Design review of the part built by this model. Coordinates are the model's own, in mm. Coordinates: 2 decimals unless noted, no trailing zeros. Loops run counter-clockwise (first coordinate to the right, second up) from the corner with the lowest first, then second, coordinate; pieces in that order, holes last. Notation, with made-up numbers: (-7.75, -32.75) -> (23.25, -32.75) arc R22 cw to (23.25, 5.25) -> close; hole circle Ø3 at (-12, 18.5). An arc over 180 degrees is marked (long way). Answer in a Markdown table with one row per item.
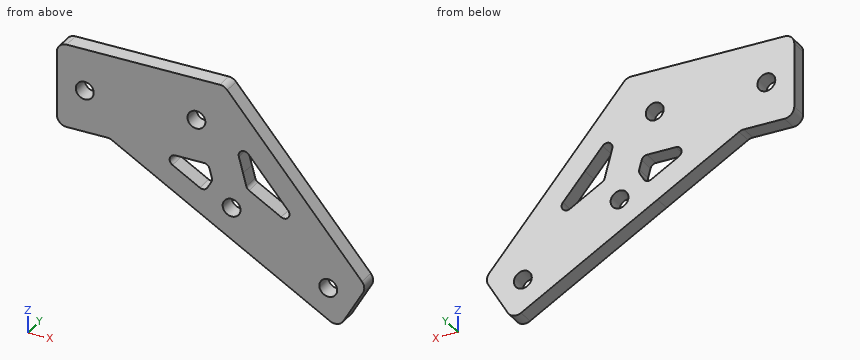
```python
from build123d import *

# Parameters (mm, degrees)
SKETCH_2_R          = 1.6
EXTRUDE_1_DEPTH     = 1.5
CUT_EXTRUDE_1_DEPTH = 3
FILLET_1_R          = 1
FILLET_2_R          = 1.75


with BuildPart() as part:
    # ｽｹｯﾁ2 → ﾎﾞｽ - 押し出し1 (new, symmetric)
    with BuildSketch(Plane(origin=(0, 0, 0), x_dir=(1, 0, 0), z_dir=(0, 1, 0))):
        Polygon((24.47, 8.660254038), (9.47, 0), (0, 0), (0, -15), (30, -15), (55.450762114, 15), (50.450762114, 23.660254038), align=None)
        with Locations(Location((48.620635095, 16.830127019, 0), (0, 0, 270))):
            Circle(SKETCH_2_R, mode=Mode.SUBTRACT)
        with Locations(Location((25, -7.5, 0), (0, 0, 270))):
            Circle(SKETCH_2_R, mode=Mode.SUBTRACT)
        with Locations(Location((31.300127019, 6.830127019, 0), (0, 0, 270))):
            Circle(SKETCH_2_R, mode=Mode.SUBTRACT)
        with Locations(Location((5, -7.5, 0), (0, 0, 270))):
            Circle(SKETCH_2_R, mode=Mode.SUBTRACT)
    extrude(amount=EXTRUDE_1_DEPTH, both=True)

    # ｽｹｯﾁ3 → ｶｯﾄ - 押し出し1 (cut)
    with BuildSketch(Plane(origin=(0, 1.5, 0), x_dir=(1, 0, 0), z_dir=(0, 1, 0))):
        Polygon((26.47, 5.196152423), (17.47, 0), (27.140628594, 0), (27.879009742, 2.755675961), align=None)
        Polygon((33.352285677, 0), (37.479868618, 0), (45.169472556, 9.064094706), (34.062793268, 2.651650429), align=None)
        Polygon((31.44676478, -7.111500799), (37.479868618, 0), (33.352285677, 0), align=None)
    extrude(amount=-CUT_EXTRUDE_1_DEPTH, mode=Mode.SUBTRACT)

    # ﾌｨﾚｯﾄ1
    fillet_1_edges = [part.edges().sort_by_distance(p)[0] for p in [
        (27.879009742, 0, -2.755675961),
        (27.140628594, 0, 0),
        (17.47, 0, 0),
        (26.47, 0, -5.196152423),
        (34.062793268, 0, -2.651650429),
        (45.169472556, 0, -9.064094706),
        (31.44676478, 0, 7.111500799),
    ]]
    fillet(fillet_1_edges, radius=FILLET_1_R)

    # ﾌｨﾚｯﾄ2
    fillet_2_edges = [part.edges().sort_by_distance(p)[0] for p in [
        (50.450762114, 0, -23.660254038),
        (55.450762114, 0, -15),
        (30, 0, 15),
        (0, 0, 15),
        (0, 0, 0),
        (9.47, 0, 0),
    ]]
    fillet(fillet_2_edges, radius=FILLET_2_R)


solid = part.part
```
(1) Take a section at A-A on x = 5. Give the boundary of the cut face in (y, z), and give its area (3 significant figures).
Evaluation:
| item | result |
|---|---|
| outline | (-1.5, 0) -> (1.5, 0) -> (1.5, 5.9) -> (-1.5, 5.9) -> close; (-1.5, 9.1) -> (1.5, 9.1) -> (1.5, 15) -> (-1.5, 15) -> close |
| area | 35.4 mm² |
(2) Take a section at B-B on z = 7.5. Give the boundary of the cut face in (x, y).
Evaluation:
| item | result |
|---|---|
| outline | (0, -1.5) -> (3.4, -1.5) -> (3.4, 1.5) -> (0, 1.5) -> close; (6.6, -1.5) -> (23.4, -1.5) -> (23.4, 1.5) -> (6.6, 1.5) -> close; (26.6, -1.5) -> (36.36, -1.5) -> (36.36, 1.5) -> (26.6, 1.5) -> close |
(3) For pin 1 (1.5 mm diameter, centred on x = 24.5, y = -1, fed in from -Z); pin 2 (0.9 mm diameter, centred on x = 4.5, y = 0.5, fed in from -Z); pin 3 (1.5 mm diameter, centred on x = 24, y = 0.5, fed in from -Z), all flat-tipped, find the tip position at first contact; note any pin that passes through.
Evaluation:
| item | result |
|---|---|
| pin 1 | stops at z = -9.11 |
| pin 2 | stops at z = 0 |
| pin 3 | stops at z = -8.82 |
(4) Take a section at C-C on y = -0.7. Count the separate pieces of the cut face and the enclosed holes in it, and give its area (3 significant figures).
Evaluation:
| item | result |
|---|---|
| separate pieces | 1 |
| enclosed holes | 6 |
| area | 933 mm² |
(5) To check wall thickness, follow probe 1 along X at (y, z) = (0.15, 7.5); probe 2 along Z at (x, y) = (8.5, 1.1); probe 3 along X at (y, z) = (0.5, 7). State the ranges of each line that lie inside material, in increasing order.
Evaluation:
| item | result |
|---|---|
| probe 1 | x = 0 to 3.4, 6.6 to 23.4, 26.6 to 36.36 |
| probe 2 | z = 0 to 15 |
| probe 3 | x = 0 to 3.48, 6.52 to 23.48, 26.52 to 36.79 |
(6) Take a section at D-D on z = -12.5. Give the boundary of the cut face in (x, y), and give its area (3 significant figures).
Evaluation:
| item | result |
|---|---|
| outline | (31.12, -1.5) -> (53.33, -1.5) -> (53.33, 1.5) -> (31.12, 1.5) -> close |
| area | 66.6 mm² |
